Geometry check sheet. Reference: the model listing, model coordinates, mm. Round coordinates to 2 decimals unless told otherwise and drop trailing zeros. Write each loop counter-clockwise with the first axis right and the second up, starting at its lowest first coordinate (ties: lowest second). Pieces come first, ordered by that corner, then holes. Notation, with made-up numbers: (26.25, -19.5) - (42.25, -19.5) arc R34 ccw to (42.25, 11.5) - close; hole circle Ø1 at (83.25, 73.5). An arc over 180 degrees is marked (long way). Return JSON: item names as keys, results as strings. Group by question number.
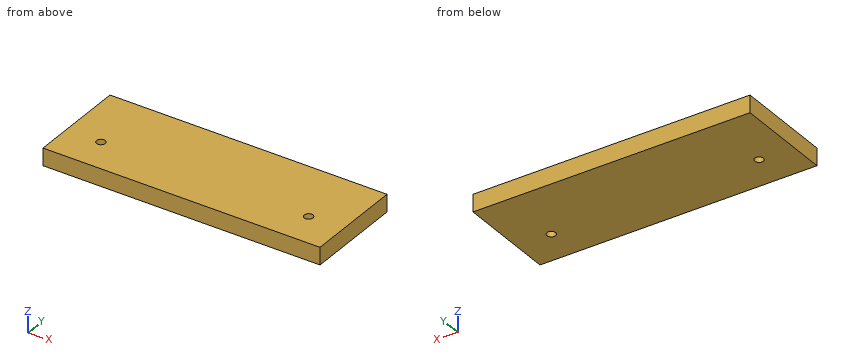
from build123d import *

# Parameters (mm, degrees)
F0_W     = 203.2
F0_H     = 73.025
F1_DEPTH = 12.7
F3_DEPTH = 25.4


with BuildPart() as f1:
    # F0 (on Top) → F1 (new body)
    with BuildSketch(Plane.XY):
        with Locations((-101.6, 36.5125)):
            Rectangle(F0_W, F0_H)
    extrude(amount=F1_DEPTH)

    # F2 (on face) → F3 (cut)
    with BuildSketch(Plane.XY.offset(12.7)):
        with BuildLine():
            Line((-177.8, 25.4), (-180.975, 25.4))
            ThreePointArc((-180.975, 25.4), (-177.8, 22.225), (-174.625, 25.4))
            Line((-174.625, 25.4), (-177.8, 25.4))
        make_face()
        with BuildLine():
            ThreePointArc((-174.625, 25.4), (-177.8, 28.575), (-180.975, 25.4))
            Line((-180.975, 25.4), (-177.8, 25.4))
            Line((-177.8, 25.4), (-174.625, 25.4))
        make_face()
        with BuildLine():
            ThreePointArc((-28.575, 25.4), (-25.4, 22.225), (-22.225, 25.4))
            Line((-22.225, 25.4), (-25.4, 25.4))
            Line((-25.4, 25.4), (-28.575, 25.4))
        make_face()
        with BuildLine():
            Line((-25.4, 25.4), (-22.225, 25.4))
            ThreePointArc((-22.225, 25.4), (-25.4, 28.575), (-28.575, 25.4))
            Line((-28.575, 25.4), (-25.4, 25.4))
        make_face()
    extrude(amount=-F3_DEPTH, mode=Mode.SUBTRACT)


solid = f1.part
1. Section check B-B (y = 25.4). Enter the section's corners in (x, z) (3 decimals), and give its area (3 significant figures).
2. Material ranges on line 1 along Y through (x, z) = (-25.4, 6.25) (3 decimals), recorded low to high.
3. Depth check by flat-ended pin: pin 1 Ø2 at (x, z) = (-151.5, 11) entering from -Y. Enter the tip coordinate at first touch or a pass-through.
4. Section check A-A (x = -177.8). Enter the section's corners in (y, z) (3 decimals), and give its area (3 significant figures).
Result sheet:
{
 "1": {"outline": "(-203.2, 0) - (-180.975, 0) - (-180.975, 12.7) - (-203.2, 12.7) - close; (-174.625, 0) - (-28.575, 0) - (-28.575, 12.7) - (-174.625, 12.7) - close; (-22.225, 0) - (0, 0) - (0, 12.7) - (-22.225, 12.7) - close", "area": "2,420 mm²"},
 "2": {"line 1": "y = 0 to 22.225, 28.575 to 73.025"},
 "3": {"pin 1": "stops at y = 0"},
 "4": {"outline": "(0, 0) - (22.225, 0) - (22.225, 12.7) - (0, 12.7) - close; (28.575, 0) - (73.025, 0) - (73.025, 12.7) - (28.575, 12.7) - close", "area": "847 mm²"}
}
